Could you check a few things on this model? Use its own coordinates, in mm. Face numbers are marked on the shaded views. A direction names the side the tool comes from. Coordinates: 2 decimals unless noted, no trailing zeros. Write each loop counter-clockwise with the first axis right and the second up, starting at its lowest first coordinate (ties: lowest second). Pieces come first, ordered by that corner, then holes.
```python
from build123d import *

# Parameters (mm, degrees)
SKETCH1_R            = 6.5
BOSS_EXTRUDE1_DEPTH  = 10
CUT_EXTRUDE1_DEPTH   = 2
FILLET1_R            = 2
FILLET1_OF_MIRROR4_R = 2
FILLET2_R            = 50
SKETCH3_R            = 3
CUT_EXTRUDE2_DEPTH   = 10
SKETCH4_R            = 15
CUT_EXTRUDE3_DEPTH   = 14
CHAMFER1_SIZE        = 1
CUT_EXTRUDE4_START   = -6
SKETCH5_R            = 16
CUT_EXTRUDE4_DEPTH   = 1.5


with BuildPart() as part:
    # Sketch1 → Boss-Extrude1 (new, symmetric)
    with BuildSketch(Plane(origin=(0, 0, 0), x_dir=(0, 0, -1), z_dir=(1, 0, 0))):
        with BuildLine():
            Line((-46, -11.205497968), (46, -11.205497968))
            Line((46, -11.205497968), (46, 3.794502032))
            Line((46, 3.794502032), (30, 68.794502032))
            Line((30, 68.794502032), (30, 120.794502032))
            Line((30, 120.794502032), (25, 125.794502032))
            Line((25, 125.794502032), (18.33030278, 125.794502032))
            ThreePointArc((18.33030278, 125.794502032), (16.33030278, 126.211926337), (14.664242224, 127.394502032))
            ThreePointArc((14.664242224, 127.394502032), (0, 133.794502032), (-14.664242224, 127.394502032))
            ThreePointArc((-14.664242224, 127.394502032), (-16.33030278, 126.211926337), (-18.33030278, 125.794502032))
            Line((-18.33030278, 125.794502032), (-25, 125.794502032))
            Line((-25, 125.794502032), (-30, 120.794502032))
            Line((-30, 120.794502032), (-30, 68.794502032))
            Line((-30, 68.794502032), (-46, 3.794502032))
            Line((-46, 3.794502032), (-46, -11.205497968))
        make_face()
        with Locations((0, 113.794502032)):
            Circle(SKETCH1_R, mode=Mode.SUBTRACT)
    extrude(amount=BOSS_EXTRUDE1_DEPTH, both=True)

    # Sketch2 → Cut-Extrude1 (cut, symmetric)
    with BuildSketch(Plane(origin=(10, 0, 0), x_dir=(0, 0, -1), z_dir=(1, 0, 0))):
        with BuildLine():
            Line((13, 88.794502032), (-13, 88.794502032))
            ThreePointArc((-13, 88.794502032), (-16.535533906, 87.330035938), (-18, 83.794502032))
            Line((-18, 83.794502032), (-18, 73.402647758))
            ThreePointArc((-18, 73.402647758), (-18.363636327, 67.383395202), (-19.449256053, 61.451695402))
            Line((-19.449256053, 61.451695402), (-30.886080209, 14.989597267))
            ThreePointArc((-30.886080209, 14.989597267), (-29.966452179, 10.710306527), (-26.031005815, 8.794502032))
            Line((-26.031005815, 8.794502032), (26.031005815, 8.794502032))
            ThreePointArc((26.031005815, 8.794502032), (29.966452179, 10.710306527), (30.886080209, 14.989597267))
            Line((30.886080209, 14.989597267), (19.449256053, 61.451695402))
            ThreePointArc((19.449256053, 61.451695402), (18.363636327, 67.383395202), (18, 73.402647758))
            Line((18, 73.402647758), (18, 83.794502032))
            ThreePointArc((18, 83.794502032), (16.535533906, 87.330035938), (13, 88.794502032))
        make_face()
    cut_extrude1 = extrude(amount=CUT_EXTRUDE1_DEPTH, both=True, mode=Mode.SUBTRACT)

    # Fillet1
    fillet1_edges = [part.edges().sort_by_distance(p)[0] for p in [
        (8, 38.220646335, 25.167668131),
        (8, 67.383395202, 18.363636327),
        (8, 78.598574895, 18),
        (8, 87.330035938, 16.535533906),
        (8, 88.794502032, 0),
        (8, 87.330035938, -16.535533906),
        (8, 78.598574895, -18),
        (8, 67.383395202, -18.363636327),
        (8, 38.220646335, -25.167668131),
        (8, 10.710306527, -29.966452179),
        (8, 8.794502032, 0),
        (8, 10.710306527, 29.966452179),
    ]]
    fillet(fillet1_edges, radius=FILLET1_R - 0.0001)  # a hair under: the kernel refuses the full size

    # Mirror4: Cut-Extrude1 across plane
    add(cut_extrude1.mirror(Plane(origin=(0, 0, 0), x_dir=(0, 0, 1), z_dir=(1, 0, 0))), mode=Mode.SUBTRACT)

    # Fillet1 of Mirror4
    fillet1_of_mirror4_edges = [part.edges().sort_by_distance(p)[0] for p in [
        (-8, 38.220646335, 25.167668131),
        (-8, 67.383395202, 18.363636327),
        (-8, 78.598574895, 18),
        (-8, 87.330035938, 16.535533906),
        (-8, 88.794502032, 0),
        (-8, 87.330035938, -16.535533906),
        (-8, 78.598574895, -18),
        (-8, 67.383395202, -18.363636327),
        (-8, 38.220646335, -25.167668131),
        (-8, 10.710306527, -29.966452179),
        (-8, 8.794502032, 0),
        (-8, 10.710306527, 29.966452179),
    ]]
    fillet(fillet1_of_mirror4_edges, radius=FILLET1_OF_MIRROR4_R - 0.0001)  # a hair under: the kernel refuses the full size

    # Fillet2
    fillet2_edges = [part.edges().sort_by_distance(p)[0] for p in [
        (0, 68.794502032, 30),
        (0, 68.794502032, -30),
    ]]
    fillet(fillet2_edges, radius=FILLET2_R)

    # Sketch3 → Cut-Extrude2 (cut)
    with BuildSketch(Plane.XZ.offset(11.205497968)):
        with Locations(Location((0, 30, 0), (0, 0, 270))):
            Circle(SKETCH3_R)
        with Locations(Location((0, -30, 0), (0, 0, 270))):
            Circle(SKETCH3_R)
    extrude(amount=-CUT_EXTRUDE2_DEPTH, mode=Mode.SUBTRACT)

    # Sketch4 → Cut-Extrude3 (cut)
    with BuildSketch(Plane.ZY.offset(10)):
        with Locations((0, 113.794502032)):
            Circle(SKETCH4_R)
    extrude(amount=-CUT_EXTRUDE3_DEPTH, mode=Mode.SUBTRACT)

    # Chamfer1
    chamfer1_edges = [part.edges().sort_by_distance(p)[0] for p in [
        (-10, 113.794502032, -15),
    ]]
    chamfer(chamfer1_edges, length=CHAMFER1_SIZE)

    # Sketch5 → Cut-Extrude4 (cut)
    with BuildSketch(Plane.ZY.offset(10).offset(CUT_EXTRUDE4_START)):
        with Locations((0, 113.794502032)):
            Circle(SKETCH5_R)
    extrude(amount=CUT_EXTRUDE4_DEPTH, mode=Mode.SUBTRACT)


solid = part.part
```
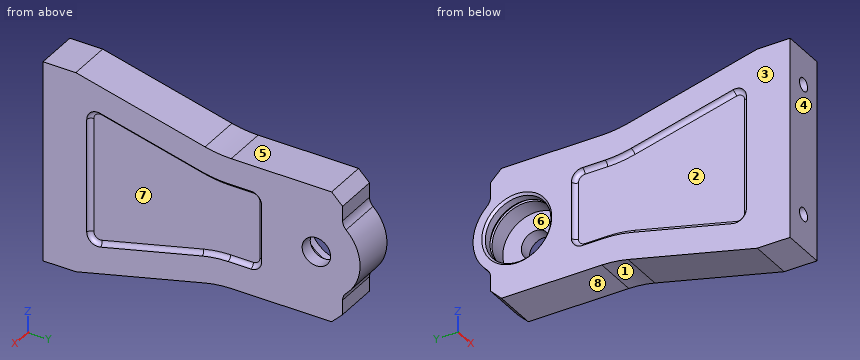
1. Please list where these lines run through material, in increasing order: line 1 along Y through (x, z) = (5.85, 0); line 2 along Y through (x, z) = (-8.3, 0); line 3 along X through (y, z) = (29, 3.5).
Verdict:
line 1: y = -11.21 to 107.29, 120.29 to 133.79
line 2: y = -11.21 to 9.74, 87.85 to 98.79, 128.79 to 133.79
line 3: x = -8 to 8
2. On a 3-axis mill with a long thin cutter (end or side, diameter ignored), from which of +Z, -Z, +X, -X, +Y, -Y can I reach the whole of each face in a straight line? I mean the marked faces 4, 5, 6, 7 and 8. Say none if no direction works.
Verdict:
face 4: +Z, -Z, +X, -X, -Y
face 5: +Z, +X, -X, +Y
face 6: -X
face 7: +X
face 8: -Z, +X, -X, +Y
3. I want a section at B-B on x = 0. Please give me the cut outline in (y, z).
Verdict:
outline: (-11.21, -46) - (3.79, -46) - (62.91, -31.45) arc R50 cw to (74.86, -30) - (120.79, -30) - (125.79, -25) - (125.79, -18.33) arc R5 cw to (127.39, -14.66) arc R20 ccw to (127.39, 14.66) arc R5 cw to (125.79, 18.33) - (125.79, 25) - (120.79, 30) - (74.86, 30) arc R50 cw to (62.91, 31.45) - (3.79, 46) - (-11.21, 46) - (-11.21, 33) - (-1.21, 33) - (-1.21, 27) - (-11.21, 27) - (-11.21, -27) - (-1.21, -27) - (-1.21, -33) - (-11.21, -33) - close; hole circle Ø30 at (113.79, 0)
4. I want a section at C-C on y = 92.5. Please give me the cut outline in (x, z), plus the area to 3 significant figures.
Verdict:
outline: (-10, -30) - (10, -30) - (10, 30) - (-10, 30) - close
area: 1,200 mm2
5. If we mould it in two halves opening along Z, with no side actions, what happens to the marked faces 1, 2 and 3? For each: pulls with the +Z half, pulls with the -Z half, needs draft (parallel to the pull), parting line crosses it, or undercut.
Verdict:
face 1: pulls with the -Z half
face 2: undercut
face 3: needs draft
6. For pin 1 (10 mm diameter, centred on x = -5.5, y = 90, fed in from -Z); pin 2 (5 mm diameter, centred on x = 3.5, z = 5, fed in from +Y); pin 3 (3 mm diameter, centred on x = 7.5, y = 20.5, fed in from -Z); pin 4 (11.5 mm diameter, centred on y = 113.79, z = 0, fed in from -X), each with a flat end and sliding along its axis, tell me the tip position at first contact or that it passes through.
Verdict:
pin 1: stops at z = -30
pin 2: stops at y = 133.64
pin 3: stops at z = -42.26
pin 4: passes through
